from build123d import *

# Parameters (mm, degrees)
SKETCH1_R           = 13.25
SKETCH1_R_2         = 2.05
BOSS_EXTRUDE1_DEPTH = 2
SKETCH2_R           = 2
BOSS_EXTRUDE2_DEPTH = 2
BOSS_EXTRUDE3_DEPTH = 2
BOSS_EXTRUDE4_DEPTH = 2
SKETCH5_W           = 7
SKETCH5_H           = 5
CUT_EXTRUDE1_DEPTH  = 2
SKETCH6_W           = 20
SKETCH6_H           = 5
CUT_EXTRUDE2_DEPTH  = 2
FILLET1_R           = 3
SKETCH8_W           = 25
SKETCH8_H           = 8
BOSS_EXTRUDE5_DEPTH = 2


with BuildPart() as part:
    # Sketch1 → Boss-Extrude1 (new body)
    with BuildSketch(Plane(origin=(0, 0, 0), x_dir=(0, 0, -1), z_dir=(1, 0, 0))):
        with BuildLine():
            Line((-13, 21.5), (13, 21.5))
            ThreePointArc((13, 21.5), (20.071067812, 18.571067812), (23, 11.5))
            Line((23, 11.5), (23, -21.5))
            Line((23, -21.5), (-23, -21.5))
            Line((-23, -21.5), (-23, 11.5))
            ThreePointArc((-23, 11.5), (-20.071067812, 18.571067812), (-13, 21.5))
        make_face()
        Circle(SKETCH1_R, mode=Mode.SUBTRACT)
        with Locations((0, 17.5)):
            Circle(SKETCH1_R_2, mode=Mode.SUBTRACT)
        with Locations((17.5, 0)):
            Circle(SKETCH1_R_2, mode=Mode.SUBTRACT)
        with Locations((0, -17.5)):
            Circle(SKETCH1_R_2, mode=Mode.SUBTRACT)
        with Locations((-17.5, 0)):
            Circle(SKETCH1_R_2, mode=Mode.SUBTRACT)
    extrude(amount=BOSS_EXTRUDE1_DEPTH)

    # Sketch2 → Boss-Extrude2 (add)
    # profile 1 of 2: a face of its own
    with BuildSketch(Plane.XZ.offset(21.5)):
        Polygon((-5, 23), (-25, 23), (-25, 47), (-5, 47), (-5, 28), (2, 28), (2, 23), align=None)
        with Locations(Location((-20, 35, 0), (0, 0, 270))):
            Circle(SKETCH2_R, mode=Mode.SUBTRACT)
        with Locations(Location((-10, 35, 0), (0, 0, 90))):
            Circle(SKETCH2_R, mode=Mode.SUBTRACT)
    # profile 2 of 2: a face of its own
    with BuildSketch(Plane.XZ.offset(21.5)):
        Polygon((2, -23), (-5, -23), (-25, -23), (-25, -47), (-5, -47), (-5, -28), (2, -28), align=None)
        with Locations(Location((-10, -35, 0), (0, 0, 270))):
            Circle(SKETCH2_R, mode=Mode.SUBTRACT)
        with Locations(Location((-20, -35, 0), (0, 0, 90))):
            Circle(SKETCH2_R, mode=Mode.SUBTRACT)
    extrude(amount=-BOSS_EXTRUDE2_DEPTH)

    # Sketch3 → Boss-Extrude3 (add)
    with BuildSketch(Plane(origin=(0, 0, -23), x_dir=(-1, 0, 0), z_dir=(0, 0, -1))):
        Polygon((-2, 11.5), (0, 11.5), (25, -19.5), (15, -19.5), (0, -0.9), (-2, -0.9), align=None)
    extrude(amount=BOSS_EXTRUDE3_DEPTH)

    # Sketch4 → Boss-Extrude4 (add)
    with BuildSketch(Plane.XY.offset(23)):
        Polygon((2, 11.5), (0, 11.5), (-25, -19.5), (-15, -19.5), (0, -0.9), (2, -0.9), align=None)
    extrude(amount=BOSS_EXTRUDE4_DEPTH)

    # Sketch5 → Cut-Extrude1 (cut)
    with BuildSketch(Plane.XZ.offset(21.5)):
        with Locations((-1.5, 25.5)):
            Rectangle(SKETCH5_W, SKETCH5_H)
        with Locations((-1.5, -25.5)):
            Rectangle(SKETCH5_W, SKETCH5_H)
    extrude(amount=-CUT_EXTRUDE1_DEPTH, mode=Mode.SUBTRACT)

    # Sketch6 → Cut-Extrude2 (cut)
    with BuildSketch(Plane(origin=(0, -19.5, 0), x_dir=(1, 0, 0), z_dir=(0, 1, 0))):
        with Locations((-15, 44.5)):
            Rectangle(SKETCH6_W, SKETCH6_H)
        with Locations((-15, -44.5)):
            Rectangle(SKETCH6_W, SKETCH6_H)
    extrude(amount=-CUT_EXTRUDE2_DEPTH, mode=Mode.SUBTRACT)

    # Fillet1
    fillet1_edges = [part.edges().sort_by_distance(p)[0] for p in [
        (-5, -20.5, -42),
        (-25, -20.5, -42),
        (-25, -20.5, 42),
        (-5, -20.5, 42),
    ]]
    fillet(fillet1_edges, radius=FILLET1_R)

    # Sketch8 → Boss-Extrude5 (add)
    with BuildSketch(Plane.XZ.offset(21.5)):
        with Locations((-12.5, 19)):
            Rectangle(SKETCH8_W, SKETCH8_H)
        with Locations((-12.5, -19)):
            Rectangle(SKETCH8_W, SKETCH8_H)
    extrude(amount=-BOSS_EXTRUDE5_DEPTH)


solid = part.part
Read the model definition and answer for the solid it produces. Units are mm, in the model's axes. A direction names the side the tool comes from. Give positions to 0.01 mm unless a question says otherwise; leave off trailing zeros. Loops run counter-clockwise (first coordinate to the right, second up) from the corner with the lowest first, then second, coordinate; pieces in that order, holes last. Notation, with made-up numbers: (-16.5, 26.5) - (1.5, 26.5) arc R19 cw to (1.5, 30.5) - close; hole circle Ø8 at (7.25, -37). An arc over 180 degrees is marked (long way). Answer as CSV lines item,"result". Start each with the question number.
1) Find section C-C (y = -6). Write down the section's boundary in (x, z).
2) Find section A-A (x = -17). Write down the section's boundary in (y, z), then the cut area to 3 significant figures.
3) Each of these flat-tipped pins is pushed along its axis until it touches: pin 1 Ø21.5 at (y, z) = (-1, 8.5) entering from -X; pin 2 Ø3.5 at (y, z) = (-17.5, 0) entering from -X; pin 3 Ø1 at (x, z) = (1, -24) entering from -Y; pin 4 Ø8 at (x, y) = (-5, -4) entering from +Z. Where does it stop, or does it pass through?
4) Find section D-D (z = 17.5). Write down the section's boundary in (x, y), then the cut area to 3 significant figures.
5) Straight lines are drawn through the part: L1, parallel to X at y = -20.2, z = -35; L2, parallel to Z at x = -0.75, y = -1.5; L3, parallel to Y at x = 1.1, z = 0. For each, find the intervals that lie inside material, in ascending order. Write a range as from..to.
6) Which of the six approach directions +Z, -Z, +X, -X, +Y, -Y give full straight-line access (tool end or side, diameter ignored) to faces 1 (the face through (-7.605, -10.33, -23.986)), 2 (the face through (-10, -6, -25)), 3 (the face through (-9.399, -20.514, -36.908)), 4 (the face through (-10, -6, 25)), 5 (the face through (0.986, -15.467, 0.267))?
7) Determine the mould class of faces 6 (the face through (-25, -21, 27)), 7 (the face through (0.99, 18.65, -19.99)), 8 (the face through (-11, -7, -23)) for opening direction Z: released by +Z, released by -Z, zero draft, split by the parting line, or undercut.
8) Find section B-B (z = -35). Write down the section's boundary in (x, y), then the cut area to 3 significant figures.
Findings below:
1,outline,"(-14.11, -25) - (-4.11, -25) - (-4.11, -23) - (-14.11, -23) - close; (-14.11, 23) - (-4.11, 23) - (-4.11, 25) - (-14.11, 25) - close; (0, -23) - (2, -23) - (2, -11.81) - (0, -11.81) - close; (0, 11.81) - (2, 11.81) - (2, 23) - (0, 23) - close"
2,outline,"(-21.5, -42) - (-19.5, -42) - (-19.5, -25) - (-9.58, -25) - (-9.58, -23) - (-19.5, -23) - (-19.5, -15) - (-21.5, -15) - close; (-21.5, 15) - (-19.5, 15) - (-19.5, 23) - (-9.58, 23) - (-9.58, 25) - (-19.5, 25) - (-19.5, 42) - (-21.5, 42) - close"
2,area,"148 mm^2"
3,pin 1,"x = 0"
3,pin 2,"through"
3,pin 3,"y = -0.9"
3,pin 4,"z = 25"
4,outline,"(-25, -21.5) - (2, -21.5) - (2, -2.05) - (0, -2.05) - (0, -19.5) - (-25, -19.5) - close; (0, 2.05) - (2, 2.05) - (2, 20.43) - (0, 20.43) - close"
4,area,"126 mm^2"
5,L1,"-25..-22, -18..-12, -8..-5"
5,L2,"-25..-23, 23..25"
5,L3,"-21.5..-19.55, -15.45..-13.25, 13.25..15.45, 19.55..21.5"
6,face 1,"+Z, -Z, +X"
6,face 2,"-Z, +X, -X, +Y"
6,face 3,"+Y, -Y"
6,face 4,"+Z, +X, -X, +Y"
6,face 5,"+X, -X"
7,face 6,"zero draft"
7,face 7,"released by -Z"
7,face 8,"undercut"
8,outline,"(-25, -21.5) - (-22, -21.5) - (-22, -19.5) - (-25, -19.5) - close; (-18, -21.5) - (-12, -21.5) - (-12, -19.5) - (-18, -19.5) - close; (-8, -21.5) - (-5, -21.5) - (-5, -19.5) - (-8, -19.5) - close"
8,area,"24.0 mm^2"
